Can you work these out from the model? Positions are in its coordinate system, mm. Give positions to 0.01 mm unless a question says otherwise; leave off trailing zeros. Loops run counter-clockwise (first coordinate to the right, second up) from the corner with the lowest first, then second, coordinate; pieces in that order, holes last. Notation, with made-up numbers: (79, 81) - (130, 81) arc R16 cw to (130, 96) - close; hole circle Ø10 at (-4.75, 85). An arc over 180 degrees is marked (long way). Answer in a Markdown table with one row per item.
from build123d import *

# Parameters (mm, degrees)
SKETCH_1_W             = 300
SKETCH_1_H             = 70
EXTRUDE_1_DEPTH        = 2.5
SKETCH_2_R             = 1.5
SKETCH_2_R_2           = 6
CUT_EXTRUDE_1_DEPTH    = 155.04950503
PATTERN_LINEAR_1_COUNT = 9
PATTERN_LINEAR_1_PITCH = 30.48
CUT_EXTRUDE_2_DEPTH    = 10


with BuildPart() as part:
    # 草图1 → 凸台-拉伸1 (new body)
    with BuildSketch(Plane.XY):
        Rectangle(SKETCH_1_W, SKETCH_1_H)
    extrude(amount=EXTRUDE_1_DEPTH)

    # 草图2 → 切除-拉伸1 (cut, through all)
    with BuildSketch(Plane.XY.offset(2.5)):
        with Locations((-118.24, -32)):
            Circle(SKETCH_2_R)
        with Locations((-118.24, 30)):
            Circle(SKETCH_2_R)
        with Locations((-118.24, 17)):
            Circle(SKETCH_2_R_2)
        with BuildLine():
            Line((-104.060660172, -33.060660172), (-141.060660172, 3.939339828))
            ThreePointArc((-141.060660172, 3.939339828), (-141.060660172, 6.060660172), (-138.939339828, 6.060660172))
            Line((-138.939339828, 6.060660172), (-101.939339828, -30.939339828))
            ThreePointArc((-101.939339828, -30.939339828), (-101.939339828, -33.060660172), (-104.060660172, -33.060660172))
        make_face()
    cut_extrude_1 = extrude(amount=-CUT_EXTRUDE_1_DEPTH, mode=Mode.SUBTRACT)

    # 阵列(线性)1: 切除-拉伸1 ×9
    with Locations(*[(i * PATTERN_LINEAR_1_PITCH, 0, 0) for i in range(1, PATTERN_LINEAR_1_COUNT)]):
        add(cut_extrude_1, mode=Mode.SUBTRACT)

    # 草图3 → 切除-拉伸2 (cut)
    with BuildSketch(Plane.XY.offset(2.5)):
        Polygon((-11.56, 35), (-11.56, 13), (26.16, -24.72), (26.16, -35), (-150, -35), (-150, 35), align=None)
    extrude(amount=-CUT_EXTRUDE_2_DEPTH, mode=Mode.SUBTRACT)


solid = part.part
Q1. If we mould it in two halves opening along X, with no side actions, what happens to faces 1 (the face through (7.04, -5.6, 1.27)), 2 (the face through (100.843, 18.802, 1.268)), 3 (the face through (68, 0, 0))? For each: released by +X, released by -X, zero draft, split by the parting line, or undercut.
Checked values:
| item | result |
|---|---|
| face 1 | released by -X |
| face 2 | undercut |
| face 3 | zero draft |
Q2. Imagine slicing it at A-A, the plane x = 34.16. Write out the boundary of the cut face in (y, z), and give its area (3 significant figures).
Checked values:
| item | result |
|---|---|
| outline | (-35, 0) - (-33.5, 0) - (-33.5, 2.5) - (-35, 2.5) - close; (-30.5, 0) - (-18.88, 0) - (-18.88, 2.5) - (-30.5, 2.5) - close; (-14.64, 0) - (11, 0) - (11, 2.5) - (-14.64, 2.5) - close; (23, 0) - (28.5, 0) - (28.5, 2.5) - (23, 2.5) - close; (31.5, 0) - (35, 0) - (35, 2.5) - (31.5, 2.5) - close |
| area | 119 mm² |
Q3. Imagine slicing it at B-B, the plane y = -5.5. Write out the boundary of the cut face in (x, z), and give its area (3 significant figures).
Checked values:
| item | result |
|---|---|
| outline | (6.94, 0) - (20.78, 0) - (20.78, 2.5) - (6.94, 2.5) - close; (25.02, 0) - (51.26, 0) - (51.26, 2.5) - (25.02, 2.5) - close; (55.5, 0) - (81.74, 0) - (81.74, 2.5) - (55.5, 2.5) - close; (85.98, 0) - (112.22, 0) - (112.22, 2.5) - (85.98, 2.5) - close; (116.46, 0) - (150, 0) - (150, 2.5) - (116.46, 2.5) - close |
| area | 315 mm² |
Q4. Imagine slicing it at C-C, the plane z = 0.5. Count the separate pieces of the cut face and the enclosed holes in it, and give its area (3 significant figures).
Checked values:
| item | result |
|---|---|
| separate pieces | 1 |
| enclosed holes | 18 |
| area | 8,920 mm² |
Q5. For pin 1 (5 mm diameter, centred on x = 3.68, y = 30, fed in from -Z); pin 2 (1.2 mm diameter, centred on y = -31, z = 1, fed in from -X), each with a flat end and sliding along its axis, tell me the tip position at first contact or that it passes through.
Checked values:
| item | result |
|---|---|
| pin 1 | stops at z = 0 |
| pin 2 | stops at x = 26.16 |
Q6. Imagine slicing it at D-D, the plane y = 21.5. Write out the boundary of the cut face in (x, z).
Checked values:
| item | result |
|---|---|
| outline | (-11.56, 0) - (-0.29, 0) - (-0.29, 2.5) - (-11.56, 2.5) - close; (7.65, 0) - (30.19, 0) - (30.19, 2.5) - (7.65, 2.5) - close; (38.13, 0) - (60.67, 0) - (60.67, 2.5) - (38.13, 2.5) - close; (68.61, 0) - (91.15, 0) - (91.15, 2.5) - (68.61, 2.5) - close; (99.09, 0) - (121.63, 0) - (121.63, 2.5) - (99.09, 2.5) - close; (129.57, 0) - (150, 0) - (150, 2.5) - (129.57, 2.5) - close |
Q7. If I drill on line 1 (X direction, y = -30, z = 0.8); line 2 (X direction, y = 16, z = 0.3); line 3 (Y direction, x = 3.68, z = 1.15), over which ranges is the centre line in solid material (lowest first)? Write a range as [from, to].
Checked values:
| item | result |
|---|---|
| line 1 | x = [26.16, 45.28], [49.52, 75.76], [80, 106.24], [110.48, 136.72], [140.96, 150] |
| line 2 | x = [-11.56, -2.24], [9.6, 28.24], [40.08, 58.72], [70.56, 89.2], [101.04, 119.68], [131.52, 150] |
| line 3 | y = [-2.24, 11], [23, 28.5], [31.5, 35] |
